Work out the finished part from the listing and answer in its coordinate system (mm). Give positions to 0.01 mm unless a question says otherwise; leave off trailing zeros. Order: outer loops, then holes, each group sorted by start corner. A loop starts at its lowest first (then second) coordinate and runs counter-clockwise, first axis right, second up. Notation, with made-up numbers: (-30, -16) - (-15, -16) arc R29 cw to (-15, 6) - close; hole circle Ø11 at (82, 35). An arc over 180 degrees is marked (long way). Write each question's results on one line, items separated by ' | '.
from build123d import *

# Parameters (mm, degrees)
BOSS_EXTRUDE1_DEPTH   = 10
BODY_MOVE_COPY1_ANGLE = 120


with BuildPart() as part:
    # Sketch1 → Boss-Extrude1 (new body)
    with BuildSketch(Plane(origin=(0, 0, 0), x_dir=(1, 0, 0), z_dir=(0, 1, 0))):
        with BuildLine():
            Line((-10, 0), (10, 0))
            Line((10, 0), (10, 100))
            ThreePointArc((10, 100), (0, 110), (-10, 100))
            Line((-10, 100), (-10, 0))
        make_face()
        with BuildLine():
            ThreePointArc((1.5875, 98.4125), (0, 97.75493597), (-1.5875, 98.4125))
            ThreePointArc((-1.5875, 98.4125), (-2.24506403, 100), (-1.5875, 101.5875))
            ThreePointArc((-1.5875, 101.5875), (0, 102.24506403), (1.5875, 101.5875))
            ThreePointArc((1.5875, 101.5875), (2.074168707, 100.859148809), (2.24506403, 100))
            ThreePointArc((2.24506403, 100), (2.074168707, 99.140851191), (1.5875, 98.4125))
        make_face(mode=Mode.SUBTRACT)
    extrude(amount=BOSS_EXTRUDE1_DEPTH)


with BuildPart() as part_1:
    # Body-Move/Copy1: moved
    add(part.part.moved(Location((0, 0, 0))).rotate(Axis((-1.666666667, 3.333333333, -1.666666667), (0.5773502691894747, 0.5773502691901298, 0.5773502691892728)), BODY_MOVE_COPY1_ANGLE))


with BuildPart() as part_2:
    # Body-Move/Copy2: moved
    add(part_1.part.moved(Location((100, -5, 0))))


solid = part_2.part
1. A cutting plane is placed at B-B, the plane z = 3.25. Write down the section's boundary in (x, y), then the cut area to 3 significant figures.
Answer list:
outline: (0, -10) - (100, -10) - (100, 10) - (0, 10) arc R10 ccw to start; hole circle Ø4.49 at (0, 0) | area: 2,140 mm^2
2. A cutting plane is placed at C-C, the plane y = 6. Write down the section's boundary in (x, z), then the cut area to 3 significant figures.
Answer list:
outline: (-8, -5) - (100, -5) - (100, 5) - (-8, 5) - close | area: 1,080 mm^2
3. Straight lines are drawn through the part: line 1 (X direction, y = 1, z = -0.25); line 2 (X direction, y = -5, z = 0.75); line 3 (X direction, y = -5.5, z = 2.25). For each, find the intervals that lie inside material, in ascending order. Write a range as [from, to].
Answer list:
line 1: [-9.95, -2.01], [2.01, 100] | line 2: [-8.66, 100] | line 3: [-8.35, 100]
4. A cutting plane is placed at A-A, the plane y = 0. Write down the section's boundary in (x, z), then the cut area to 3 significant figures.
Answer list:
outline: (-10, -5) - (-2.25, -5) - (-2.25, 5) - (-10, 5) - close; (2.25, -5) - (100, -5) - (100, 5) - (2.25, 5) - close | area: 1,060 mm^2
